from build123d import *

# Parameters (mm, degrees)
SKETCH1_W                                           = 17
SKETCH1_H                                           = 20
BOSS_EXTRUDE1_DEPTH                                 = 2
SKETCH2_R                                           = 1.5
BOSS_EXTRUDE2_DEPTH                                 = 2.8
FILLET1_R                                           = 5.5
FILLET1_OF_MIRROR1_R                                = 5.5
CSK_FOR_M3_COUNTERSUNK_FLAT_HEAD_SCREW1_D           = 3.4
CSK_FOR_M3_COUNTERSUNK_FLAT_HEAD_SCREW1_DEPTH       = 7
CSK_FOR_M3_COUNTERSUNK_FLAT_HEAD_SCREW1_CSINK_D     = 6.3
CSK_FOR_M3_COUNTERSUNK_FLAT_HEAD_SCREW1_CSINK_ANGLE = 90
CSK_FOR_M3_COUNTERSUNK_FLAT_HEAD_SCREW1_TIP         = 1.021463052
BOSS_EXTRUDE3_DEPTH                                 = 2
FILLET2_R                                           = 7
BOSS_EXTRUDE4_DEPTH                                 = 20
FILLET3_R                                           = 9
FILLET4_R                                           = 9
FILLET5_R                                           = 1


# Some blends are built 0.0001 mm under size
with BuildPart() as part:
    # Sketch1 → Boss-Extrude1 (new body)
    with BuildSketch(Plane.XY):
        with Locations((-3.5, 0)):
            Rectangle(SKETCH1_W, SKETCH1_H)
    extrude(amount=BOSS_EXTRUDE1_DEPTH)

    # Sketch2 → Boss-Extrude2 (add)
    with BuildSketch(Plane(origin=(0, 10, 0), x_dir=(1, 0, 0), z_dir=(0, 1, 0))):
        with BuildLine():
            Line((5, 0), (-5, 0))
            Line((-5, 0), (-5, 5.5))
            ThreePointArc((-5, 5.5), (0, 10.5), (5, 5.5))
            Line((5, 5.5), (5, 0))
        make_face()
        with Locations(Location((0, 5.5, 0), (0, 0, 270))):
            Circle(SKETCH2_R, mode=Mode.SUBTRACT)
    boss_extrude2 = extrude(amount=-BOSS_EXTRUDE2_DEPTH)

    # Fillet1
    fillet1_edges = [part.edges().sort_by_distance(p)[0] for p in [
        (-5, 8.6, 0),
    ]]
    fillet(fillet1_edges, radius=FILLET1_R - 0.0001)  # a hair under: the kernel refuses the full size

    # Mirror1: Boss-Extrude2 across plane
    add(boss_extrude2.mirror(Plane.ZX))

    # Fillet1 of Mirror1
    fillet1_of_mirror1_edges = [part.edges().sort_by_distance(p)[0] for p in [
        (-5, -8.6, 0),
    ]]
    fillet(fillet1_of_mirror1_edges, radius=FILLET1_OF_MIRROR1_R - 0.0001)  # a hair under: the kernel refuses the full size

    # CSK for M3 Countersunk Flat Head Screw1
    with Locations(Plane(origin=(0, -10, 0), x_dir=(-1, 0, 0), z_dir=(0, -1, 0))):
        with Locations((0, 5.5)):
            CounterSinkHole(CSK_FOR_M3_COUNTERSUNK_FLAT_HEAD_SCREW1_D / 2, CSK_FOR_M3_COUNTERSUNK_FLAT_HEAD_SCREW1_CSINK_D / 2, depth=CSK_FOR_M3_COUNTERSUNK_FLAT_HEAD_SCREW1_DEPTH, counter_sink_angle=CSK_FOR_M3_COUNTERSUNK_FLAT_HEAD_SCREW1_CSINK_ANGLE)
            with Locations((0, 0, -(CSK_FOR_M3_COUNTERSUNK_FLAT_HEAD_SCREW1_DEPTH + CSK_FOR_M3_COUNTERSUNK_FLAT_HEAD_SCREW1_TIP / 2))):  # 118° drill point
                Cone(0, CSK_FOR_M3_COUNTERSUNK_FLAT_HEAD_SCREW1_D / 2, CSK_FOR_M3_COUNTERSUNK_FLAT_HEAD_SCREW1_TIP, mode=Mode.SUBTRACT)

    # Sketch5 → Boss-Extrude3 (add)
    with BuildSketch(Plane.XY.offset(2)):
        with BuildLine():
            Line((-12, 10), (-12, -10))
            ThreePointArc((-12, -10), (-20, 0), (-12, 10))
        make_face()
    extrude(amount=-BOSS_EXTRUDE3_DEPTH)

    # Fillet2
    fillet2_edges = [part.edges().sort_by_distance(p)[0] for p in [
        (-12, -10, 1),
        (-12, 10, 1),
    ]]
    fillet(fillet2_edges, radius=FILLET2_R)

    # Sketch6 → Boss-Extrude4 (add)
    with BuildSketch(Plane(origin=(0, 10, 0), x_dir=(1, 0, 0), z_dir=(0, 1, 0))):
        with BuildLine():
            Line((2.239887411, -2), (4.367153275, -0.888811472))
            ThreePointArc((4.367153275, -0.888811472), (20.461428056, -10.333152259), (36, 0))
            ThreePointArc((36, 0), (37.588145554, 0.59815859), (38.186304144, -0.989986964))
            ThreePointArc((38.186304144, -0.989986964), (20.528836027, -12.73220544), (2.239887411, -2))
        make_face()
    extrude(amount=-BOSS_EXTRUDE4_DEPTH)

    # Fillet3
    # the kernel refuses this fillet: 9 mm, written as the material it adds along each edge
    with BuildSketch(Plane(origin=(5, -10, 2), x_dir=(0, 0, -1), z_dir=(0, 1, 0))) as fillet3_piece_1_section:
        with BuildLine():
            CenterArc((3.066869404, -9), FILLET3_R, 90, 46.064417531)
            ThreePointArc((-3.414213733, -2.755357386), (-1.793300325, -1.270874802), (0, 0))
            Line((0, 0), (3.066869404, 0))
        make_face()
    fillet3_piece_1 = extrude(amount=20, mode=Mode.PRIVATE)
    fillet3_piece_1 = split(fillet3_piece_1, bisect_by=Plane(origin=(4.921450274, -8.6, 0), z_dir=(0, 0, -1)), keep=Keep.TOP, mode=Mode.PRIVATE)
    fillet3_piece_1 = split(fillet3_piece_1, bisect_by=Plane(origin=(4.921450274, -7.2, -0.505403298), z_dir=(0, -1, 0)), keep=Keep.TOP, mode=Mode.PRIVATE)
    add(fillet3_piece_1)
    with BuildSketch(Plane(origin=(5, -10, 2), x_dir=(0, 0, -1), z_dir=(0, 1, 0))) as fillet3_piece_2_section:
        with BuildLine():
            CenterArc((3.066869404, -9), FILLET3_R, 90, 46.064417531)
            ThreePointArc((-3.414213733, -2.755357386), (-1.793300325, -1.270874802), (0, 0))
            Line((0, 0), (3.066869404, 0))
        make_face()
    fillet3_piece_2 = extrude(amount=20, mode=Mode.PRIVATE)
    fillet3_piece_2 = split(fillet3_piece_2, bisect_by=Plane(origin=(5.669505966, -8.6, 0), z_dir=(0, 0, 1)), keep=Keep.TOP, mode=Mode.PRIVATE)
    fillet3_piece_2 = split(fillet3_piece_2, bisect_by=Plane(origin=(5.669505966, -7.2, 2.571944176), z_dir=(0, -1, 0)), keep=Keep.TOP, mode=Mode.PRIVATE)
    add(fillet3_piece_2)
    with BuildSketch(Plane(origin=(5, -10, 2), x_dir=(0, 0, -1), z_dir=(0, 1, 0))) as fillet3_piece_3_section:
        with BuildLine():
            CenterArc((3.066869404, -9), FILLET3_R, 90, 46.064417531)
            ThreePointArc((-3.414213733, -2.755357386), (-1.793300325, -1.270874802), (0, 0))
            Line((0, 0), (3.066869404, 0))
        make_face()
    fillet3_piece_3 = extrude(amount=20, mode=Mode.PRIVATE)
    fillet3_piece_3 = split(fillet3_piece_3, bisect_by=Plane(origin=(5.669505966, 0, 0), z_dir=(0, 0, 1)), keep=Keep.TOP, mode=Mode.PRIVATE)
    fillet3_piece_3 = split(fillet3_piece_3, bisect_by=Plane(origin=(5.669505966, 7.2, 2.571944176), z_dir=(0, -1, 0)), keep=Keep.TOP, mode=Mode.PRIVATE)
    fillet3_piece_3 = split(fillet3_piece_3, bisect_by=Plane(origin=(5.669505966, -7.2, 2.571944176), z_dir=(0, 1, 0)), keep=Keep.TOP, mode=Mode.PRIVATE)
    add(fillet3_piece_3)
    with BuildSketch(Plane(origin=(5, -10, 2), x_dir=(0, 0, -1), z_dir=(0, 1, 0))) as fillet3_piece_4_section:
        with BuildLine():
            CenterArc((3.066869404, -9), FILLET3_R, 90, 46.064417531)
            ThreePointArc((-3.414213733, -2.755357386), (-1.793300325, -1.270874802), (0, 0))
            Line((0, 0), (3.066869404, 0))
        make_face()
    fillet3_piece_4 = extrude(amount=20, mode=Mode.PRIVATE)
    fillet3_piece_4 = split(fillet3_piece_4, bisect_by=Plane(origin=(4.921450274, 8.6, 0), z_dir=(0, 0, -1)), keep=Keep.TOP, mode=Mode.PRIVATE)
    fillet3_piece_4 = split(fillet3_piece_4, bisect_by=Plane(origin=(4.921450274, 7.2, -0.505403298), z_dir=(0, 1, 0)), keep=Keep.TOP, mode=Mode.PRIVATE)
    add(fillet3_piece_4)
    with BuildSketch(Plane(origin=(5, -10, 2), x_dir=(0, 0, -1), z_dir=(0, 1, 0))) as fillet3_piece_5_section:
        with BuildLine():
            CenterArc((3.066869404, -9), FILLET3_R, 90, 46.064417531)
            ThreePointArc((-3.414213733, -2.755357386), (-1.793300325, -1.270874802), (0, 0))
            Line((0, 0), (3.066869404, 0))
        make_face()
    fillet3_piece_5 = extrude(amount=20, mode=Mode.PRIVATE)
    fillet3_piece_5 = split(fillet3_piece_5, bisect_by=Plane(origin=(5.669505966, 8.6, 0), z_dir=(0, 0, 1)), keep=Keep.TOP, mode=Mode.PRIVATE)
    fillet3_piece_5 = split(fillet3_piece_5, bisect_by=Plane(origin=(5.669505966, 7.2, 2.571944176), z_dir=(0, 1, 0)), keep=Keep.TOP, mode=Mode.PRIVATE)
    add(fillet3_piece_5)

    # Fillet4
    fillet4_edges = [part.edges().sort_by_distance(p)[0] for p in [
        (2.239887411, 0, 2),
    ]]
    fillet(fillet4_edges, radius=FILLET4_R)

    # Fillet5
    fillet5_edges = [part.edges().sort_by_distance(p)[0] for p in [
        (5.063457622, 0, 0),
    ]]
    fillet(fillet5_edges, radius=FILLET5_R)


solid = part.part
Work out the finished part from the listing and answer in its coordinate system (mm). A direction names the side the tool comes from. Round coordinates to 2 decimals unless told otherwise and drop trailing zeros. Write each loop counter-clockwise with the first axis right and the second up, starting at its lowest first coordinate (ties: lowest second). Pieces come first, ordered by that corner, then holes.
1) Straight lines are drawn through the part: line 1 (X direction, y = 8.3, z = -5.5); line 2 (X direction, y = -6.75, z = 1); line 3 (Z direction, x = -14.5, y = 3). For each, find the intervals that lie inside material, in ascending order.
2) Given pin 1 Ø3.5 at (x, z) = (0, -5.5) entering from -Y; pin 2 Ø1.4 at (y, z) = (9.5, -2.5) entering from +X; pin 3 Ø1.5 at (x, y) = (32, -3) entering from -Z; pin 4 Ø3 at (y, z) = (1.5, 1.5) entering from +X, each flat-ended and moving along its own axis, determine where each tip first touches the part or whether it passes through.
3) A cutting plane is placed at B-B (y = 2.75). Give the vertices of the cut face in (x, z) (3 decimals).
4) A cutting plane is placed at D-D (x = -14.5). Give the vertices of the cut face in (y, z), plus the area to 3 significant figures.
5) The mould has two halves that part along Y. Classify faces 5 (the flat face through (-0.8, -7.2, -3.5)), 6 (the flat face through (6, 10, 5)), 7 (the cylindrical face through (1.26, -0.14, 2.85)), 8 (the cylindrical face through (-20, 0, 1)): pulls with the +Y half, pulls with the -Y half, needs draft (parallel to the pull), parting line crosses it, or undercut.
6) A tool of negligible diameter and unlimited length cuts with its end or side. For faces 1 (the cylindrical face through (6.04, -0.14, 3.13)), 2 (the flat face through (-8, 0, 0)), 3 (the flat face through (5, 9, -3)), 4 (the flat face through (-11, 0, 2)), from which of +Z, -Z, +X, -X, +Y, -Y can it reach the whole face along a straight path? Write none if from no direction.
7) A cutting plane is placed at A-A (x = 0). Give the vertices of the cut face in (y, z), plus the area to 3 significant figures.
8) A cutting plane is placed at C-C (x = 34). Give the vertices of the cut face in (y, z).
Completed:
1. line 1: x = -5 to -1.5, 1.5 to 5
1. line 2: x = -17.46 to 5.24, 35.51 to 38.18
1. line 3: z = 0 to 2
2. pin 1: stops at y = -8.6
2. pin 2: stops at x = 5
2. pin 3: stops at z = 4.84
2. pin 4: stops at x = 38.29
3. outline: (-19.624, 0) - (4.216, 0) arc R1 ccw to (5.194, 0.793) arc R9 cw to (7.755, 5.414) arc R17.6 cw to (36, 0) arc R1.2 ccw to (38.186, 0.99) arc R20 ccw to (4.43, 5.333) arc R9 cw to (-2.562, 2) - (-19.624, 2) - close
4. outline: (-9.08, 0) - (9.08, 0) - (9.08, 2) - (-9.08, 2) - close
4. area: 36.3 mm2
5. face 5: undercut
5. face 6: pulls with the +Y half
5. face 7: needs draft
5. face 8: parting line crosses it
6. face 1: -Z, +Y, -Y
6. face 2: -Z, -X
6. face 3: -Z, +X, +Y, -Y
6. face 4: +Z, -X, +Y, -Y
7. outline: (-10, -10.5) - (-7.2, -10.5) - (-7.2, -7.2) - (-8.55, -7.2) - (-10, -8.65) - close; (-10, -2.35) - (-8.55, -3.8) - (-7.2, -3.8) - (-7.2, 0) - (7.2, 0) - (7.2, -4) - (10, -4) - (10, 2.37) - (-10, 2.37) - close; (7.2, -10.5) - (10, -10.5) - (10, -7) - (7.2, -7) - close
7. area: 86.2 mm2
8. outline: (-10, 3.36) - (10, 3.36) - (10, 6.99) - (-10, 6.99) - close
